CAD build for the part. Positions are in the model's coordinates, mm. Round coordinates to 2 decimals unless told otherwise and drop trailing zeros. Write each loop counter-clockwise with the first axis right and the second up, starting at its lowest first coordinate (ties: lowest second). Pieces come first, ordered by that corner, then holes. Notation, with made-up numbers: (-11.5, -30) -> (29.5, -30) arc R29 cw to (29.5, 9) -> close; hole circle Ø6 at (13.5, 14.25). An arc over 180 degrees is marked (long way). Put each result on its own line as item: value. Start each with the question number.
1. Drill centre lines: line 1 (Y direction, x = 0, z = -2.5); line 2 (Z direction, x = -9.5, y = -8.75); line 3 (Y direction, x = 0.5, z = -2.25). Where is each one in solid material? Low to high. Write a range as from..to.
2. Flat gauge pins, fed straight in: P1, Ø10, axis at x = 4, z = -4.5, coming from the +Y side; P2, Ø1.8, axis at x = -10, z = 10, coming from the +Y side (3 decimals); P3, Ø1.5, axis at x = 11, y = -10, coming from the -Z side; P4, Ø6, axis at y = -3.5, z = -4, coming from the -X side. Where does each tip first touch, or does it go through?
3. Pull direction X, two halves, no side cores. Call faces 1 (the cylindrical face through (11.2, -7.4, 9.1)), 2 (the flat face through (0, -7, -14.5)), 3 (the cylindrical face through (-12, -7, -9)), 4 (the flat face through (15, -7, 5)): pulls with the +X half, pulls with the -X half, needs draft (parallel to the pull), parting line crosses it, or undercut.
4. Saw through at C-C on x = 0. List the corners of the cut face in (y, z), and give its area (3 significant figures).
5. Saw through at D-D on z = 7.75. List the corners of the cut face in (x, y).
6. Saw through at B-B on y = -11. List the corners of the cut face in (x, z).
7. Saw through at A-A on y = -4. List the corners of the cut face in (x, z), and give its area (3 significant figures).
from build123d import *

# Parameters (mm, degrees)
F1_DEPTH = 15
F2_R     = 1.5
F3_DEPTH = 25
F4_R     = 5
F5_R     = 2.5
F6_DEPTH = 29.501


with BuildPart() as f1:
    # F0 (on Front) → F1 (new body)
    with BuildSketch(Plane.XZ):
        with BuildLine():
            Line((15, 0), (15, 15))
            Line((15, 15), (0, 15))
            ThreePointArc((0, 15), (10.606602, 10.606602), (15, 0))
        make_face()
        with BuildLine():
            ThreePointArc((-15, 0), (-10.606602, 10.606602), (0, 15))
            Line((0, 15), (-15, 15))
            Line((-15, 15), (-15, 0))
        make_face()
        with BuildLine():
            ThreePointArc((15, 0), (10.606602, 10.606602), (0, 15))
            ThreePointArc((0, 15), (-10.606602, 10.606602), (-15, 0))
            ThreePointArc((-15, 0), (-11.887148, -9.148536), (-3.840573, -14.5))
            Line((-3.840573, -14.5), (3.840573, -14.5))
            ThreePointArc((3.840573, -14.5), (11.887148, -9.148536), (15, 0))
        make_face()
    extrude(amount=F1_DEPTH)

    # F2 (on face) → F3 (cut)
    with BuildSketch(Plane(origin=(0, 0, 0), x_dir=(-1, 0, 0), z_dir=(0, 1, 0))):
        with Locations((10, 10)):
            Circle(F2_R)
        with Locations((-10, 10)):
            Circle(F2_R)
    extrude(amount=-F3_DEPTH, mode=Mode.SUBTRACT)

    # F4
    f4_edges = [f1.edges().sort_by_distance(p)[0] for p in [
        (-15, -7.5, 15),
        (15, -7.5, 15),
    ]]
    fillet(f4_edges, radius=F4_R)

    # F5 (on face) → F6 (cut, through all)
    with BuildSketch(Plane.XY.offset(15)):
        with Locations((0, -4)):
            Circle(F5_R)
    extrude(amount=-F6_DEPTH, mode=Mode.SUBTRACT)


solid = f1.part
Return value:
1. line 1: y = -15..-6.5, -1.5..0
1. line 2: z = -11.61..8.59, 11.41..15
1. line 3: y = -15..-6.45, -1.55..0
2. P1: stops at y = 0
2. P2: passes through
2. P3: stops at z = -10.95
2. P4: stops at x = -14.97
3. face 1: undercut
3. face 2: needs draft
3. face 3: pulls with the -X half
3. face 4: pulls with the +X half
4. outline: (-15, -14.5) -> (-6.5, -14.5) -> (-6.5, 15) -> (-15, 15) -> close; (-1.5, -14.5) -> (0, -14.5) -> (0, 15) -> (-1.5, 15) -> close
4. area: 295 mm^2
5. outline: (-15, -15) -> (15, -15) -> (15, 0) -> (-15, 0) -> close; hole circle Ø5 at (0, -4)
6. outline: (-15, 0) arc R15 ccw to (-3.84, -14.5) -> (3.84, -14.5) arc R15 ccw to (15, 0) -> (15, 10) arc R5 ccw to (10, 15) -> (-10, 15) arc R5 ccw to (-15, 10) -> close; hole circle Ø3 at (-10, 10); hole circle Ø3 at (10, 10)
7. outline: (-15, 0) arc R15 ccw to (-3.84, -14.5) -> (-2.5, -14.5) -> (-2.5, 15) -> (-10, 15) arc R5 ccw to (-15, 10) -> close; (2.5, -14.5) -> (3.84, -14.5) arc R15 ccw to (15, 0) -> (15, 10) arc R5 ccw to (10, 15) -> (2.5, 15) -> close; hole circle Ø3 at (-10, 10); hole circle Ø3 at (10, 10)
7. area: 628 mm^2
